Read the model definition and answer for the solid it produces. Units are mm, in the model's axes. Coordinates: 2 decimals unless noted, no trailing zeros. Order: outer loops, then holes, each group sorted by start corner. A loop starts at its lowest first (then second) coordinate and runs counter-clockwise, first axis right, second up. Notation, with made-up numbers: M 30.5,78 L 69.5,78 A27 ccw 69.5,111 Z; hole C 31.5,38.5 d8. An arc over 180 degrees is marked long. Write each question's results on one line, items separated by ' | '.
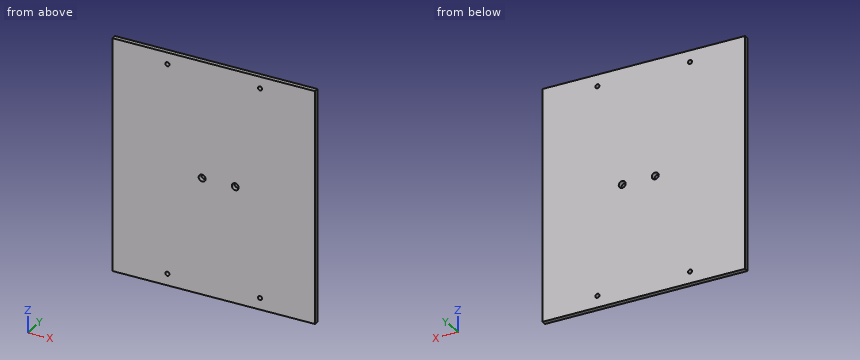
```python
from build123d import *

# Parameters (mm, degrees)
SKETCH1_W             = 222.25
SKETCH1_H             = 254
BOSS_EXTRUDE1_DEPTH   = 5.08
SKETCH2_R             = 3.81
CUT_EXTRUDE2_DEPTH    = 6.08
F_8_CLEARANCE_HOLE1_D = 4.4958


with BuildPart() as part:
    # Sketch1 → Boss-Extrude1 (new body)
    with BuildSketch(Plane(origin=(0, 0, 0), x_dir=(1, 0, 0), z_dir=(0, 1, 0))):
        Rectangle(SKETCH1_W, SKETCH1_H)
    extrude(amount=BOSS_EXTRUDE1_DEPTH)

    # Sketch2 → Cut-Extrude2 (cut, through all)
    with BuildSketch(Plane(origin=(0, 0, 0), x_dir=(1, 0, 0), z_dir=(0, 1, 0))):
        with Locations((-12.7, 0)):
            Circle(SKETCH2_R)
        with Locations((23.622, 0)):
            Circle(SKETCH2_R)
    extrude(amount=CUT_EXTRUDE2_DEPTH, mode=Mode.SUBTRACT)

    # #8 Clearance Hole1 (through all)
    with Locations(Plane(origin=(0, 0, 0), x_dir=(-1, 0, 0), z_dir=(0, -1, 0))):
        with Locations((50.8, -114.3), (-50.8, -114.3), (-50.8, 114.3), (50.8, 114.3)):
            Hole(F_8_CLEARANCE_HOLE1_D / 2)


solid = part.part
```
(1) Straight lines are drawn through the part: line 1 (Z direction, x = -50.8, y = 2.1); line 2 (X direction, y = 3.65, z = 114.3) (3 decimals); line 3 (Z direction, x = -12.7, y = 1.75). For each, find the intervals that lie inside material, in ascending order.
Conclusion:
line 1: -127 to -116.55, -112.05 to 112.05, 116.55 to 127 | line 2: -111.125 to -53.048, -48.552 to 48.552, 53.048 to 111.125 | line 3: -127 to -3.81, 3.81 to 127
(2) Given pin 1 (3.5 mm diameter, centred on x = -50.8, z = -114.3, fed in from -Y), flat-ended and moving along its own axis, determine where the tip first touches the part or whether it passes through.
Conclusion:
pin 1: through
(3) The part is cut by section B-B, the plane x = -12.7. Write down the section's boundary in (y, z), then the cut area to 3 significant figures.
Conclusion:
outline: M 0,-127 L 5.08,-127 L 5.08,-3.81 L 0,-3.81 Z; M 0,3.81 L 5.08,3.81 L 5.08,127 L 0,127 Z | area: 1,250 mm²
(4) The part is cut by section A-A, the plane z = 0. Write down the section's boundary in (x, y) (3 decimals), then the cut area to 3 significant figures.
Conclusion:
outline: M -111.125,0 L -16.51,0 L -16.51,5.08 L -111.125,5.08 Z; M -8.89,0 L 19.812,0 L 19.812,5.08 L -8.89,5.08 Z; M 27.432,0 L 111.125,0 L 111.125,5.08 L 27.432,5.08 Z | area: 1,050 mm²
